from build123d import *

# Parameters (mm, degrees)
SKETCH2_R               = 11
BOSS_EXTRUDE1_DEPTH     = 2
SKETCH3_R               = 2.5
CUT_EXTRUDE1_DEPTH      = 38.389838192
SKETCH4_W               = 8
SKETCH4_H               = 4.66
CUT_EXTRUDE2_DEPTH      = 1
CUT_EXTRUDE3_REACH      = 30.302
CUT_EXTRUDE3_END_RADIUS = 2.5
SKETCH5_R               = 2.5
SKETCH6_R               = 1.55
CUT_EXTRUDE4_DEPTH      = 27.944387171
CHAMFER1_SIZE           = 0.2
CHAMFER2_SIZE           = 0.1


with BuildPart() as part:
    # Sketch1 → Revolve1 (revolve)
    with BuildSketch(Plane(origin=(0, 0, 0), x_dir=(1, 0, 0), z_dir=(0, 1, 0))):
        with BuildLine():
            Line((-22, 4), (8.040136982, 4))
            ThreePointArc((8.040136982, 4), (9.382757902, 3.250506535), (10.725378822, 4))
            Line((10.725378822, 4), (12, 4))
            Line((12, 4), (12, 0))
            Line((12, 0), (-22, 0))
            Line((-22, 0), (-22, 4))
        make_face()
    revolve(axis=Axis((12, 0, 0), (-1, 0, 0)))

    # Sketch2 → Boss-Extrude1 (add)
    with BuildSketch(Plane(origin=(0, 0, 0), x_dir=(0, 0, -1), z_dir=(1, 0, 0))):
        Circle(SKETCH2_R)
    extrude(amount=-BOSS_EXTRUDE1_DEPTH)

    # Sketch3 → Cut-Extrude1 (cut, through all)
    with BuildSketch(Plane(origin=(12, 0, 0), x_dir=(0, 0, -1), z_dir=(1, 0, 0))):
        Circle(SKETCH3_R)
    extrude(amount=-CUT_EXTRUDE1_DEPTH, mode=Mode.SUBTRACT)

    # Sketch4 → Cut-Extrude2 (cut)
    with BuildSketch(Plane(origin=(0, 4, 0), x_dir=(1, 0, 0), z_dir=(0, 1, 0))):
        with Locations((-13.616018874, 0)):
            Rectangle(SKETCH4_W, SKETCH4_H)
    extrude(amount=-CUT_EXTRUDE2_DEPTH, mode=Mode.SUBTRACT)

    # Cut-Extrude3: up to this cylinder (the profile starts outside it)
    cut_extrude3_end = Plane(origin=(-13.804261, 0, 0), z_dir=(1, 0, 0)) * Cylinder(CUT_EXTRUDE3_END_RADIUS, 66.604, mode=Mode.PRIVATE)
    # Sketch5 → Cut-Extrude3 (cut, up to the surface)
    with BuildSketch(Plane(origin=(0, 3, 0), x_dir=(1, 0, 0), z_dir=(0, 1, 0)), mode=Mode.PRIVATE) as cut_extrude3_sk1:
        with Locations(Location((-13.804261439, 0, 0), (0, 0, 270))):
            Circle(SKETCH5_R)
    cut_extrude3_tool1 = extrude(cut_extrude3_sk1.sketch, amount=-CUT_EXTRUDE3_REACH, mode=Mode.PRIVATE) - cut_extrude3_end
    add(cut_extrude3_tool1.solids().sort_by_distance((-13.804261, 3, 0))[0], mode=Mode.SUBTRACT)

    # Sketch6 → Cut-Extrude4 (cut, through all)
    with BuildSketch(Plane(origin=(0, 0, 0), x_dir=(0, 0, -1), z_dir=(1, 0, 0))):
        with Locations((-4.776443449, 4.654384475)):
            Circle(SKETCH6_R)
        with Locations((4.654384475, 4.776443449)):
            Circle(SKETCH6_R)
        with Locations((4.776443449, -4.654384475)):
            Circle(SKETCH6_R)
        with Locations((-4.654384475, -4.776443449)):
            Circle(SKETCH6_R)
    extrude(amount=-CUT_EXTRUDE4_DEPTH, mode=Mode.SUBTRACT)

    # Chamfer1
    chamfer1_edges = [part.edges().sort_by_distance(p)[0] for p in [
        (0, 0, 4),
        (-2, 0, 4),
        (-2, 0, 11),
        (0, 0, 11),
        (-2, -4.776443449, 6.204384475),
        (0, -4.776443449, 6.204384475),
        (-2, -4.654384475, -3.226443449),
        (0, -4.654384475, -3.226443449),
        (-2, 4.776443449, -3.104384475),
        (0, 4.776443449, -3.104384475),
        (-2, 4.654384475, 6.326443449),
        (0, 4.654384475, 6.326443449),
    ]]
    chamfer(chamfer1_edges, length=CHAMFER1_SIZE)

    # Chamfer2
    chamfer2_edges = [part.edges().sort_by_distance(p)[0] for p in [
        (-22, 0, 2.5),
        (12, 0, 2.5),
        (-22, 0, 4),
        (12, 0, 4),
    ]]
    chamfer(chamfer2_edges, length=CHAMFER2_SIZE)


solid = part.part
Can you work these out from the model? Positions are in its coordinate system, mm. A direction names the side the tool comes from. Coordinates: 2 decimals unless noted, no trailing zeros. Loops run counter-clockwise (first coordinate to the right, second up) from the corner with the lowest first, then second, coordinate; pieces in that order, holes last. Notation, with made-up numbers: (88, -29) - (118, -29) arc R24 cw to (118, -3) - close; hole circle Ø2 at (3.5, -39.5). An arc over 180 degrees is marked (long way). Put each result on its own line as item: value. Start each with the question number.
Item 1: Which directions (+Z, -Z, +X, -X, +Y, -Y) give clear straight access to the entire face, cutting with the end or side of a thin tool? Please do faces 4 (the face through (-17, 3, 0)), 5 (the face through (11.321, 3.905, 0.867)), 6 (the face through (-11.912, -3.966, 0.521)).
Item 2: For pin 1 (4.5 mm diameter, centred on x = -13.8, z = 0, fed in from +Y); pin 2 (4 mm diameter, centred on y = 4.78, z = -4.65, fed in from +X); pin 3 (5 mm diameter, centred on x = -10, z = -0.5, fed in from +Y), each with a flat end and sliding along its axis, tell me the tip position at first contact or that it passes through.
Item 3: Suppose I cut it at B-B (z = 0). State how many separate pieces and enclosed holes the cut face has, and give its area (3 significant figures).
Item 4: Suppose I cut it at C-C (x = -12.5). Please give me the cut outline in (y, z).
Item 5: If I drill on line 1 along X through (y, z) = (4, -2); line 2 along X through (y, z) = (3.5, -0.5); line 3 along Z through (x, y) = (-6, 2), over which ranges is the centre line in solid material (lowest first)?
Item 6: If we mould it in two halves opening along Y, with no side actions, what happens to faces 1 (the face through (4.175, 3.905, 0.867)), 2 (the face through (-0.989, -4.311, 3.176)), 3 (the face through (-11, 3, 0))? For each: +Y half, -Y half, draft (parallel to the pull), parting line (faces both ways), or undercut.
Item 7: Suppose I cut it at A-A (x = -1). Please give me the cut outline in (y, z), and give its area (3 significant figures).
Here are the results:
1. face 4: +Y
1. face 5: +X
1. face 6: -X
2. pin 1: y = -1.09
2. pin 2: x = 0
2. pin 3: y = 4
3. separate pieces: 3
3. enclosed holes: 0
3. area: 117 mm²
4. outline: (1.3, -2.13) arc R2.5 cw (long way) to (1.3, 2.13) - (3, 2.13) - (3, 2.33) - (3.25, 2.33) arc R4 ccw (long way) to (3.25, -2.33) - (3, -2.33) - (3, -2.13) - close
5. line 1: -2 to 0
5. line 2: -22 to -17.62, -9.62 to 8.48, 10.29 to 12
5. line 3: -3.46 to -1.5, 1.5 to 3.46
6. face 1: parting line
6. face 2: undercut
6. face 3: +Y half
7. outline: circle Ø22 at (0, 0); hole circle Ø3.1 at (-4.78, 4.65); hole circle Ø3.1 at (-4.65, -4.78); hole circle Ø5 at (0, 0); hole circle Ø3.1 at (4.65, 4.78); hole circle Ø3.1 at (4.78, -4.65)
7. area: 330 mm²
